Autodesk Inventor part; units mm, degrees
ref_plane "YZ Plane" through (0, 0, 0) normal (1, 0, 0) x (0, 1, 0)
ref_plane "XZ Plane" through (0, 0, 0) normal (0, 1, 0) x (-1, 0, 0)
ref_plane "XY Plane" through (0, 0, 0) normal (0, 0, 1) x (1, 0, 0)
sketch "Skizze2" plane through (0, 0, 0) normal (0, 1, 0) x (-1, 0, 0)
  line L0 (0, 0) -> (16, 0)
  line L1 (16, 0) -> (16, 250)
  line L2 (16, 250) -> (0, 250)
  line L3 (0, 250) -> (0, 0)
  dimension "d0" = 16
  dimension "d1" = 250
extrude "Extrusion1" add sketch "Skizze2" along normal blind 10
sketch "Skizze3" plane through (0, 0, 250) normal (1, 0, 0) x (0, 0, -1)
  line L0 (250, 0) -> (0, 0)
  line L1 (250, 10) -> (0, 10)
  line L2 (10, 0) -> (12, 0)
  line L3 (12, 0) -> (12, 10)
  line L4 (12, 10) -> (10, 10)
  line L5 (10, 10) -> (10, 0)
  line L6 (0, 0) -> (0, 10)
  point P0 (10, 10)
  point P1 (12, 0)
  dimension "d4" = 2
  dimension "d5" = 10
extrude "Extrusion2" cut sketch "Skizze3" against normal blind 7.5 contours L0 L5 L1 L3
sketch "Skizze4" plane through (-16, 0, 250) normal (0, 0, 1) x (1, 0, 0)
  line L0 (0, 0) -> (16, 0)
  line L1 (16, 0) -> (16, 10)
  point P0 (13.5, 5)
  dimension "d8" = 5
  dimension "d9" = 2.5
hole "Bohrung1" at (-2.5, 5, 250) direction (0, 0, -1) diameter 4.2 depth 12
sketch "Skizze5" plane through (0, 10, 0) normal (0, 1, 0) x (1, 0, 0)
  line L0 (-16, -250) -> (0, -250)
  line L1 (-16, 0) -> (-16, -250)
  point P0 (0, 0)
  point P1 (-8, -239)
  dimension "d17" = 11
  dimension "d18" = 8
hole "Bohrung2" at (-8, 10, 239) direction (0, -1, 0) diameter 6 depth 18 tip angle 118
sketch "Skizze7" plane through (0, 10, 0) normal (0, 1, 0) x (1, 0, 0)
  circle A0 centre (-8, -9) radius 7.05
  line L0 (0, -238) -> (0, 0)
  line L1 (0, 0) -> (-16, 0)
  arc A1 (-5.1716, -238) -> (-5.1716, -240) centre (-8, -239) ccw
  dimension "d35" = 14.1
  dimension "d36" = 8
  dimension "d43" = 230
extrude "Extrusion3" cut sketch "Skizze7" against normal blind 9
sketch "Skizze9" plane through (0, 10, 0) normal (0, 1, 0) x (1, 0, 0)
  circle A0 centre (-8, -9) radius 7.05
  circle A1 centre (-8, -9) radius 6.05
  point P0 (0, 0)
  dimension "d40" = 12.1
extrude "Extrusion4" cut sketch "Skizze9" against normal through all contours A1
sketch "Skizze10" plane through (-16, 0, 250) normal (0, 0, 1) x (1, 0, 0)
  circle A0 centre (13.5, 5) radius 2.1
  point P0 (16, 0)
hole "Bohrung4" at (-2.5, 5, 250) direction (0, 0, -1) diameter 3.242 depth 18 tip angle 118
properties part number "Arm"
Geometry check sheet. Reference: the model listing, model coordinates, mm. A direction names the side the tool comes from. Coordinates: 2 decimals unless noted, no trailing zeros. Loops run counter-clockwise (first coordinate to the right, second up) from the corner with the lowest first, then second, coordinate; pieces in that order, holes last. Notation, with made-up numbers: (-35, 67) - (20, 67) arc R13 ccw to (20, 84) - close; hole circle Ø1 at (37, 37.5). An arc over 180 degrees is marked (long way). One line per item, written item: value. Start each with the question number.
(1) Mould release check, pull along X, two halves, no side actions. Record for faces 6 (the flat face through (-8, 10, 127)), 7 (the cylindrical face through (-9.312, 0.507, 14.906)), 8 (the flat face through (0, 5, 121)), 9 (the flat face through (-6, 1, 3)): released by +X, released by -X, zero draft, split by the parting line, or undercut.
(2) Material ranges on line 1 (X direction, y = 6.25, z = 9); line 2 (Y direction, x = -2.5, z = 236.6); line 3 (Z direction, x = -8, y = 3.25), recorded low to high. Write a range as [from, to].
(3) Tool access check on faces 1 (the flat face through (-2.5, 7.3, 240)), 2 (the flat face through (-16, 5, 123)), 3 (the flat face through (-8, 5, 0)), 4 (the cylindrical face through (-13.595, 5.563, 13.29)), 5 (the cylindrical face through (-0.45, 5.46, 244.93)). Record the directions out of +Z, -Z, +X, -X, +Y, -Y that give a thin tool (end or side, any length) a straight path to the whole face; none if there is none.
(4) Cross-section at A-A on z = 9. Enter the section's corners in (x, y).
(5) Depth check by flat-ended pin: P1, Ø4, axis at x = -2.5, y = 5, coming from the +Z side; P2, Ø2.5, axis at x = -2.5, y = 5, coming from the +Z side; P3, Ø3.5, axis at x = -8, z = 239, coming from the -Y side. Enter the tip coordinate at first touch or a pass-through.
(6) Cross-section at B-B on x = -8. Enter the section's corners in (y, z), plus the area to 3 significant figures.
Results below:
1. face 6: zero draft
1. face 7: undercut
1. face 8: released by +X
1. face 9: undercut
2. line 1: x = [-16, -15.05], [-0.95, 0]
2. line 2: y = [0, 3.38], [6.62, 10]
2. line 3: z = [0, 1.95], [16.05, 236], [242, 250]
3. face 1: +X, +Y, -Y
3. face 2: +Z, -Z, -X, +Y, -Y
3. face 3: -Z, +X, -X, +Y, -Y
3. face 4: +Y
3. face 5: +Z
4. outline: (-16, 0) - (-14.05, 0) - (-14.05, 1) - (-15.05, 1) - (-15.05, 10) - (-16, 10) - close; (-1.95, 0) - (0, 0) - (0, 10) - (-0.95, 10) - (-0.95, 1) - (-1.95, 1) - close
5. P1: stops at z = 238
5. P2: stops at z = 231.78
5. P3: passes through
6. outline: (0, 0) - (10, 0) - (10, 1.95) - (1, 1.95) - (1, 2.95) - (0, 2.95) - close; (0, 15.05) - (1, 15.05) - (1, 16.05) - (10, 16.05) - (10, 236) - (0, 236) - close; (0, 242) - (10, 242) - (10, 250) - (0, 250) - close
6. area: 2,300 mm2
